Autodesk Inventor part; units mm, degrees
ref_plane "YZ Plane" through (0, 0, 0) normal (1, 0, 0) x (0, 1, 0)
ref_plane "XZ Plane" through (0, 0, 0) normal (0, 1, 0) x (-1, 0, 0)
ref_plane "XY Plane" through (0, 0, 0) normal (0, 0, 1) x (1, 0, 0)
ref_plane "Arbeitsebene1" through (0, 0, 0) normal (0, 0, 1) x (1, 0, 0)
sketch "Skizze1" plane through (0, 0, 0) normal (0, 0, 1) x (1, 0, 0)
  line L0 (76.5043, -50) -> (76.5043, 50)
  arc A0 (96.5043, 50) -> (76.5043, 50) centre (86.5043, 50) ccw
  line L1 (96.5043, 50) -> (96.5043, -50)
  arc A1 (76.5043, -50) -> (96.5043, -50) centre (86.5043, -50) ccw
  line L2 (-95.8131, -50) -> (-95.8131, 50)
  arc A2 (-75.8131, 50) -> (-95.8131, 50) centre (-85.8131, 50) ccw
  line L3 (-75.8131, 50) -> (-75.8131, -50)
  arc A3 (-95.8131, -50) -> (-75.8131, -50) centre (-85.8131, -50) ccw
  line L4 (-118.5, -74.5) -> (-118.5, 74.5)
  arc A4 (-118.5, -74.5) -> (-103.5, -89.5) centre (-103.5, -74.5) ccw
  line L5 (56.1, -89.5) -> (-103.5, -89.5)
  line L6 (56.1, -83) -> (56.1, -89.5)
  arc A5 (71.1, -68) -> (56.1, -83) centre (71.1, -83) ccw
  line L7 (80.5, -68) -> (71.1, -68)
  arc A6 (95.5, -83) -> (80.5, -68) centre (80.5, -83) ccw
  line L8 (95.5, -89.5) -> (95.5, -83)
  line L9 (103.5, -89.5) -> (95.5, -89.5)
  arc A7 (103.5, -89.5) -> (118.5, -74.5) centre (103.5, -74.5) ccw
  line L10 (118.5, 74.5) -> (118.5, -74.5)
  arc A8 (118.5, 74.5) -> (103.5, 89.5) centre (103.5, 74.5) ccw
  line L11 (-103.5, 89.5) -> (103.5, 89.5)
  arc A9 (-103.5, 89.5) -> (-118.5, 74.5) centre (-103.5, 74.5) ccw
  circle A10 centre (-58.5, 18.7) radius 1.4
  circle A11 centre (-58.5, 36.552) radius 1.4
  circle A12 centre (57.5, 20.252) radius 1.4
  circle A13 centre (57.5, 35) radius 1.4
  circle A14 centre (-58.5, 8.7) radius 1.4
  circle A15 centre (-58.5, -9.152) radius 1.4
  circle A16 centre (57.5, 7.148) radius 1.4
  circle A17 centre (57.5, -7.6) radius 1.4
  circle A18 centre (103.5, 74.5) radius 1.4
  circle A19 centre (103.5, -74.5) radius 1.4
  circle A20 centre (-103.5, -74.5) radius 1.4
  circle A21 centre (-103.5, 74.5) radius 1.4
  line L12 (20.9567, 0.5738) -> (-20.9567, 0.5738)
  line L13 (-20.9567, 0.5738) -> (-20.9567, 30.6837)
  line L14 (-20.9567, 30.6837) -> (20.9567, 30.6837)
  line L15 (20.9567, 30.6837) -> (20.9567, 0.5738)
  circle A22 centre (73.1917, -22.4328) radius 1.4
  circle A23 centre (43.1917, -22.4328) radius 1.4
  circle A24 centre (13.1917, -22.4328) radius 1.4
  circle A25 centre (-16.8083, -22.4328) radius 1.4
  circle A26 centre (-46.8083, -22.4328) radius 1.4
  circle A27 centre (-102.338, -1.3) radius 1.4
  circle A28 centre (-102.338, 13.7) radius 1.4
  circle A29 centre (-102.338, 28.7) radius 1.4
  circle A30 centre (102.338, 28.7) radius 1.4
  circle A31 centre (-73.1917, -22.4328) radius 1.4
  circle A32 centre (-43.1917, -22.4328) radius 1.4
  circle A33 centre (-13.1917, -22.4328) radius 1.4
  circle A34 centre (16.8083, -22.4328) radius 1.4
  circle A35 centre (46.8083, -22.4328) radius 1.4
  circle A36 centre (102.338, -1.3) radius 1.4
  circle A37 centre (102.338, 13.7) radius 1.4
  circle A38 centre (-103.5, 74.5) radius 5
  line L16 (-116.5, 74.5) -> (-116.5, -74.5)
  arc A39 (-116.5, -74.5) -> (-103.5, -87.5) centre (-103.5, -74.5) ccw
  line L17 (-103.5, -87.5) -> (54.1, -87.5)
  line L18 (54.1, -87.5) -> (54.1, -83)
  arc A40 (71.1, -66) -> (54.1, -83) centre (71.1, -83) ccw
  line L19 (71.1, -66) -> (80.5, -66)
  arc A41 (97.5, -83) -> (80.5, -66) centre (80.5, -83) ccw
  line L20 (97.5, -83) -> (97.5, -87.5)
  line L21 (97.5, -87.5) -> (103.5, -87.5)
  arc A42 (103.5, -87.5) -> (116.5, -74.5) centre (103.5, -74.5) ccw
  line L22 (116.5, -74.5) -> (116.5, 74.5)
  arc A43 (116.5, 74.5) -> (103.5, 87.5) centre (103.5, 74.5) ccw
  line L23 (103.5, 87.5) -> (-103.5, 87.5)
  arc A44 (-103.5, 87.5) -> (-116.5, 74.5) centre (-103.5, 74.5) ccw
  line L24 (-98.5, 74.5) -> (-98.5, 87.5)
  line L25 (-103.5, 69.5) -> (-116.5, 69.5)
  circle A45 centre (-108.5, 79.5) radius 1.4
  circle A46 centre (-108.5, -79.5) radius 1.4
  circle A47 centre (108.5, 79.5) radius 1.4
  circle A48 centre (108.5, -79.5) radius 1.4
  point P0 (0, 0)
  dimension "d0" = 10
  dimension "d1" = 2
ref_plane "Arbeitsebene2" through (0, 0, 105.7) normal (0, 0, 1) x (1, 0, 0)
sketch "Skizze4" plane through (0, 0, 105.7) normal (0, 0, 1) x (1, 0, 0)
  line L0 (-98.5, 74.5) -> (-98.5, 87.5)
  circle A0 centre (-103.5, 74.5) radius 5
  line L1 (-103.5, 69.5) -> (-116.5, 69.5)
  arc A1 (-103.5, 87.5) -> (-116.5, 74.5) centre (-103.5, 74.5) ccw
  arc A2 (-103.5, 83.5) -> (-112.5, 74.5) centre (-103.5, 74.5) ccw
  line L2 (-103.5, 83.5) -> (-98.5, 83.5)
  line L3 (-112.5, 74.5) -> (-112.5, 69.5)
  point P0 (0, 0)
  dimension "d8" = 4
loft "Erhebung1" add profiles "Skizze1", "Skizze4" contours A21 | A38 | A38 L25 L16 A44 L23 L24 | A45 / all
sketch "Skizze5" plane through (-103.5, 69.5, 0) normal (0, 0, -1) x (-1, 0, 0)
  circle A0 centre (0, 5) radius 3.25
  circle A1 centre (0, 5) radius 1.4
  circle A2 centre (5, 10) radius 1.4
  point P0 (-103.5, -69.5)
extrude "Extrusion4" cut sketch "Skizze5" against normal blind 60 contours A1 | A2
fillet "Rundung1" radius 8 3 edges at (-109.864, 80.864, 105.7) (-101, 83.5, 105.7) (-112.5, 72, 105.7)
properties part number "60_Planktoscope_CornerPillars"
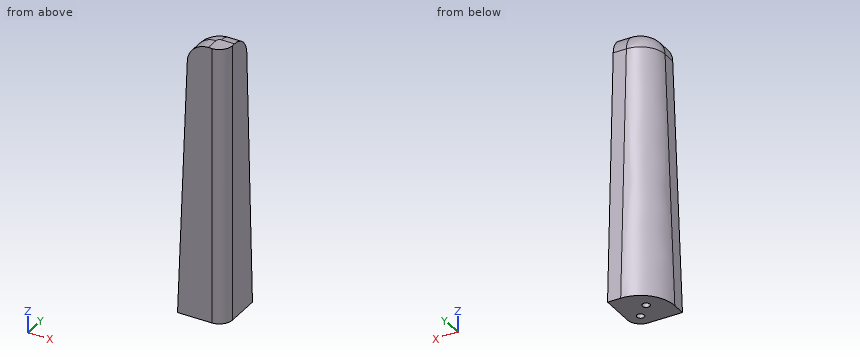
Model file for the job. Use its own axes, mm. Round coordinates to 2 decimals unless told otherwise and drop trailing zeros.
1. Band-saw the part on A-A, the plane z = 13. Count the separate pieces of the cut face and the enclosed holes in it, and give its area (3 significant figures).
Check values:
separate pieces: 1
enclosed holes: 2
area: 255 mm2
2. Drop flat-ended pins along their axis: P1, Ø5, axis at x = -111, z = 51, coming from the +Y side; P2, Ø6, axis at y = 74.5, z = 67, coming from the -X side; P3, Ø0.8, axis at x = -108, y = 80, coming from the -Z side. Give the stop position or say it passes through.
Check values:
P1: stops at y = 84.38
P2: stops at x = -114.08
P3: stops at z = 60
3. Wall check: probe 1 along Z at (x, y) = (-101.75, 76.25); probe 2 along X at (y, z) = (79.5, 39); probe 3 along Y at (x, z) = (-103.5, 47). Give the ranges that are in metal, low to high.
Check values:
probe 1: z = 0 to 105.69
probe 2: x = -113.88 to -109.9, -107.1 to -98.5
probe 3: y = 69.5 to 73.1, 75.9 to 85.72
